```python
from build123d import *

# Parameters (mm, degrees)
ESQUISSE1_W                  = 30
ESQUISSE1_H                  = 12
BOSS_EXTRU_1_DEPTH           = 20
BOSS_EXTRU_2_DEPTH           = 20
ENL_V_MAT_EXTRU_1_DEPTH      = 59.048643566
ENL_V_MAT_EXTRU_1_DEPTH_BACK = 59.048643566
ESQUISSE3_R                  = 3.5
ENL_V_MAT_EXTRU_2_DEPTH      = 63.072991509
ENL_V_MAT_EXTRU_2_DEPTH_BACK = 63.072991509
ESQUISSE4_R                  = 3
CONG_1_R                     = 3


with BuildPart() as part:
    # Esquisse1 → Boss.-Extru.1 (new body)
    with BuildSketch(Plane.XY):
        with Locations((15, 6)):
            Rectangle(ESQUISSE1_W, ESQUISSE1_H)
    extrude(amount=BOSS_EXTRU_1_DEPTH)

    # Esquisse2 → Boss.-Extru.2 (add)
    with BuildSketch(Plane.XY.offset(20)):
        Polygon((30, 0), (34.970562748, 0), (52.627416998, 17.656854249), (44.142135624, 26.142135624), (30, 12), align=None)
    extrude(amount=-BOSS_EXTRU_2_DEPTH)

    # Esquisse3 → Enlèv. mat.-Extru.1 (cut, two sides: drawn at the far end of the back side and taken through both)
    with BuildSketch(Plane(origin=(0, 12, 0), x_dir=(1, 0, 0), z_dir=(0, 1, 0)).offset(-ENL_V_MAT_EXTRU_1_DEPTH_BACK)):
        with Locations(Location((8, -10, 0), (0, 0, 270))):
            Circle(ESQUISSE3_R)
        with Locations(Location((24, -10, 0), (0, 0, 270))):
            Circle(ESQUISSE3_R)
    extrude(amount=ENL_V_MAT_EXTRU_1_DEPTH + ENL_V_MAT_EXTRU_1_DEPTH_BACK, mode=Mode.SUBTRACT)

    # Esquisse4 → Enlèv. mat.-Extru.2 (cut, two sides: drawn at the far end of the back side and taken through both)
    with BuildSketch(Plane.XY.offset(20).offset(-ENL_V_MAT_EXTRU_2_DEPTH_BACK)):
        with Locations((44.142135624, 17.656854249)):
            Circle(ESQUISSE4_R)
    extrude(amount=ENL_V_MAT_EXTRU_2_DEPTH + ENL_V_MAT_EXTRU_2_DEPTH_BACK, mode=Mode.SUBTRACT)

    # Congé1
    cong_1_edges = [part.edges().sort_by_distance(p)[0] for p in [
        (44.142135624, 26.142135624, 10),
        (52.627416998, 17.656854249, 10),
        (34.970562748, 0, 10),
        (0, 12, 10),
        (30, 12, 10),
        (0, 0, 10),
    ]]
    fillet(cong_1_edges, radius=CONG_1_R)


solid = part.part
```
Source: CAD feature listing. Evaluate the final solid. Frame: model axes, mm. A direction names the side the tool comes from. Round coordinates to 2 decimals unless told otherwise and drop trailing zeros. Write each loop counter-clockwise with the first axis right and the second up, starting at its lowest first coordinate (ties: lowest second). Pieces come first, ordered by that corner, then holes. Notation, with made-up numbers: M 47.5,83 L 92.5,83 A19 cw 92.5,93 Z; hole C 53,43 d10. An arc over 180 degrees is marked long. Answer as a JSON object with one key per item and string values. Group by question number.
(1) Reachability of faces 1 (the flat face through (48.414, 21.87, 10.14)), 2 (the flat face through (16, 12, 10)) from +Z, -Z, +X, -X, +Y, -Y: full face, straight path, thin tool, end or side. Return the list, or none.
(2) Section query A-A on z = 11. Output: boundary loops of the cut face in (x, y), then the cut area to 3 significant figures.
(3) Ray query, line 1 (Z direction, x = 8, y = 9); line 2 (X direction, y = 3.25, z = 10.75); line 3 (X direction, y = 11.25, z = 10.75). Return the intervals inside material, ascending. Write a range as [from, to].
(4) Section query D-D on z = 19. Output: boundary loops of the cut face in (x, y), then the cut area to 3 significant figures.
(5) First-contact query: pin 1 (6 mm diameter, centred on y = 16.5, z = 7.5, fed in from +X); pin 2 (6 mm diameter, centred on x = 33, z = 9, fed in from +Y); pin 3 (5.5 mm diameter, centred on x = 24, z = 10, fed in from -Y); pin 4 (9 mm diameter, centred on x = 8, z = 10, fed in from +Y). Flat tips, straight axial feed; report the tip coordinate or a pass-through.
(6) Mould query, pull axis X, two halves, no side actions, for faces 3 (the cylindrical face through (26.365, 5.916, 7.42)), 4 (the flat face through (25, 10, 0)), 5 (the cylindrical face through (34.86, 0.22, 9.86)), 6 (the cylindrical face through (29.89, 12.22, 10.14)). Classes: +X half, -X half, draft (parallel to the pull), parting line (faces both ways), or undercut.
(7) Section query C-C on y = 6.75. Output: boundary loops of the cut face in (x, z).
(8) Section query B-B on x = 8. Output: boundary loops of the cut face in (y, z).
Computed values:
{
 "1": {"face 1": "+Z, -Z, +X, +Y", "face 2": "+Z, -Z, -X, +Y"},
 "2": {"outline": "M 0,3 A3 ccw 3,0 L 4.65,0 L 4.65,12 L 3,12 A3 ccw 0,9 Z; M 11.35,0 L 20.65,0 L 20.65,12 L 11.35,12 Z; M 27.35,0 L 33.73,0 A3 ccw 35.85,0.88 L 50.51,15.54 A3 ccw 50.51,19.78 L 46.26,24.02 A3 ccw 42.02,24.02 L 30.88,12.88 A3 cw 28.76,12 L 27.35,12 Z; hole C 44.14,17.66 d6", "area": "463 mm^2"},
 "3": {"line 1": "[0, 6.5], [13.5, 20]", "line 2": "[0, 4.58], [11.42, 20.58], [27.42, 38.22]", "line 3": "[1.02, 4.58], [11.42, 20.58], [27.42, 46.22]"},
 "4": {"outline": "M 0,3 A3 ccw 3,0 L 33.73,0 A3 ccw 35.85,0.88 L 50.51,15.54 A3 ccw 50.51,19.78 L 46.26,24.02 A3 ccw 42.02,24.02 L 30.88,12.88 A3 cw 28.76,12 L 3,12 A3 ccw 0,9 Z; hole C 44.14,17.66 d6", "area": "624 mm^2"},
 "5": {"pin 1": "x = 51.38", "pin 2": "y = 18", "pin 3": "through", "pin 4": "y = 12"},
 "6": {"face 3": "undercut", "face 4": "draft", "face 5": "+X half", "face 6": "-X half"},
 "7": {"outline": "M 0,0 L 41.72,0 L 41.72,20 L 0,20 Z; hole C 8,10 d7; hole C 24,10 d7"},
 "8": {"outline": "M 0,0 L 12,0 L 12,6.5 L 0,6.5 Z; M 0,13.5 L 12,13.5 L 12,20 L 0,20 Z"}
}
